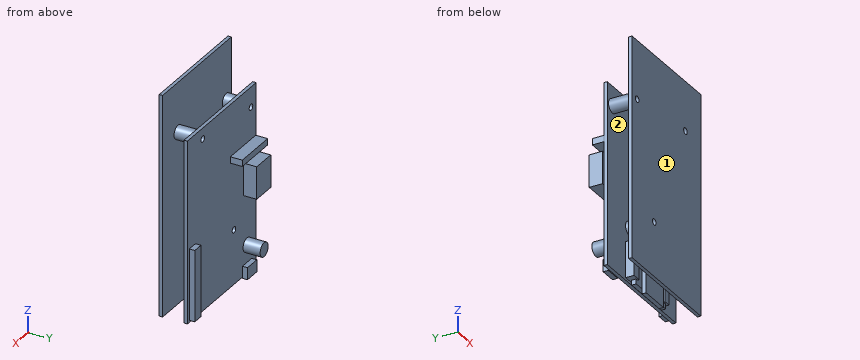
from build123d import *

# Parameters (mm, degrees)
SKETCH2_W               = 55.88
SKETCH2_H               = 85.09
FIBERGLASS_PCB_DEPTH    = 1.6
SKETCH3_W               = 7.6
SKETCH3_H               = 5.6
USB_MICRO_B_POWER_DEPTH = 2.4
SKETCH4_W               = 5
SKETCH4_H               = 33.2
BOSS_EXTRUDE3_DEPTH     = 2.6
SKETCH5_W               = 11.4
SKETCH5_H               = 15.1
BOSS_EXTRUDE4_DEPTH     = 6.15
SKETCH6_W               = 20.6
SKETCH6_H               = 2.95
BOSS_EXTRUDE5_DEPTH     = 5.6
SKETCH8_R               = 3.25
BOSS_EXTRUDE6_DEPTH     = 8
SKETCH9_W               = 28.4
SKETCH9_H               = 16.8
BOSS_EXTRUDE7_DEPTH     = 3.9
SKETCH10_W              = 24
SKETCH10_H              = 2.1
BOSS_EXTRUDE8_DEPTH     = 2.286
SKETCH11_R              = 1.45
CUT_EXTRUDE1_DEPTH      = 54.073569326
SKETCH12_R              = 3.175
BOSS_EXTRUDE9_DEPTH     = 10
SKETCH13_W              = 55.88
SKETCH13_H              = 103.09
BOSS_EXTRUDE10_DEPTH    = 1.5875
SKETCH14_R              = 1.45
CUT_EXTRUDE2_DEPTH      = 69.474424286
CUT_EXTRUDE3_DEPTH      = 0.75
SKETCH16_W              = 14.0335
SKETCH16_H              = 17.145
BOSS_EXTRUDE11_DEPTH    = 1.9685
BOSS_EXTRUDE13_REACH    = 70.474
SKETCH18_R              = 3.175
SKETCH19_R              = 1.45
CUT_EXTRUDE5_DEPTH      = 69.474424286


with BuildPart() as part:
    # Sketch2 → Fiberglass PCB (new body)
    with BuildSketch(Plane(origin=(0, 0, 0), x_dir=(1, 0, 0), z_dir=(0, 1, 0))):
        Rectangle(SKETCH2_W, SKETCH2_H)
    extrude(amount=FIBERGLASS_PCB_DEPTH)

    # Sketch3 → USB Micro-B Power (add)
    with BuildSketch(Plane(origin=(0, 1.6, 0), x_dir=(1, 0, 0), z_dir=(0, 1, 0))):
        with Locations((-20.54, 40.245)):
            Rectangle(SKETCH3_W, SKETCH3_H)
    extrude(amount=USB_MICRO_B_POWER_DEPTH)

    # Sketch4 → Boss-Extrude3 (add)
    with BuildSketch(Plane(origin=(0, 1.6, 0), x_dir=(1, 0, 0), z_dir=(0, 1, 0))):
        with Locations((23.94, 24.945)):
            Rectangle(SKETCH4_W, SKETCH4_H)
    extrude(amount=BOSS_EXTRUDE3_DEPTH)

    # Sketch5 → Boss-Extrude4 (add)
    with BuildSketch(Plane(origin=(0, 1.6, 0), x_dir=(1, 0, 0), z_dir=(0, 1, 0))):
        with Locations((-23.44, -2.505)):
            Rectangle(SKETCH5_W, SKETCH5_H)
    extrude(amount=BOSS_EXTRUDE4_DEPTH)

    # Sketch6 → Boss-Extrude5 (add)
    with BuildSketch(Plane(origin=(0, 1.6, 0), x_dir=(1, 0, 0), z_dir=(0, 1, 0))):
        with Locations((-17.26, -16.78)):
            Rectangle(SKETCH6_W, SKETCH6_H)
    extrude(amount=BOSS_EXTRUDE5_DEPTH)

    # Sketch8 → Boss-Extrude6 (add)
    with BuildSketch(Plane(origin=(0, 1.6, 0), x_dir=(1, 0, 0), z_dir=(0, 1, 0))):
        with Locations(Location((-20.54, 29.295, 0), (0, 0, 90))):
            Circle(SKETCH8_R)
    extrude(amount=BOSS_EXTRUDE6_DEPTH)

    # Sketch9 → Boss-Extrude7 (add)
    with BuildSketch(Plane.XZ):
        with Locations((1.26, -32.945)):
            Rectangle(SKETCH9_W, SKETCH9_H)
    extrude(amount=BOSS_EXTRUDE7_DEPTH)

    # Sketch10 → Boss-Extrude8 (add)
    with BuildSketch(Plane(origin=(0, 0, -41.345), x_dir=(-1, 0, 0), z_dir=(0, 0, -1))):
        with Locations((-2.097, -2.1)):
            Rectangle(SKETCH10_W, SKETCH10_H)
    extrude(amount=BOSS_EXTRUDE8_DEPTH)

    # Sketch11 → Cut-Extrude1 (cut, through all)
    with BuildSketch(Plane(origin=(0, 1.6, 0), x_dir=(1, 0, 0), z_dir=(0, 1, 0))):
        with Locations(Location((15.494, -37.465, 0), (0, 0, 270))):
            Circle(SKETCH11_R)
        with Locations(Location((-9.906, 17.145, 0), (0, 0, 270))):
            Circle(SKETCH11_R)
    extrude(amount=-CUT_EXTRUDE1_DEPTH, mode=Mode.SUBTRACT)

    # Sketch12 → Boss-Extrude9 (add)
    with BuildSketch(Plane.XZ):
        with Locations(Location((-9.906, -17.145, 0), (0, 0, 270))):
            Circle(SKETCH12_R)
        with Locations(Location((15.494, 37.465, 0), (0, 0, 270))):
            Circle(SKETCH12_R)
    extrude(amount=BOSS_EXTRUDE9_DEPTH)

    # Sketch13 → Boss-Extrude10 (add)
    with BuildSketch(Plane.XZ.offset(10)):
        with Locations((0, 9)):
            Rectangle(SKETCH13_W, SKETCH13_H)
    extrude(amount=BOSS_EXTRUDE10_DEPTH)

    # Sketch14 → Cut-Extrude2 (cut, through all)
    with BuildSketch(Plane(origin=(0, 1.6, 0), x_dir=(1, 0, 0), z_dir=(0, 1, 0))):
        with Locations(Location((-9.906, 17.145, 0), (0, 0, 270))):
            Circle(SKETCH14_R)
        with Locations(Location((15.494, -37.465, 0), (0, 0, 270))):
            Circle(SKETCH14_R)
    extrude(amount=-CUT_EXTRUDE2_DEPTH, mode=Mode.SUBTRACT)

    # Sketch15 → Cut-Extrude3 (cut)
    with BuildSketch(Plane(origin=(0, -3.9, 0), x_dir=(-1, 0, 0), z_dir=(0, -1, 0))):
        Polygon((8.7335, 41.345), (-12.412, 41.345), (-12.412, 30.12806403), (-10.16693597, 27.883), (8.7335, 27.883), align=None)
    extrude(amount=-CUT_EXTRUDE3_DEPTH, mode=Mode.SUBTRACT)

    # Sketch16 → Boss-Extrude11 (add)
    with BuildSketch(Plane.XZ.offset(3.15)):
        with Locations((1.80115, -37.4715)):
            Rectangle(SKETCH16_W, SKETCH16_H)
    extrude(amount=BOSS_EXTRUDE11_DEPTH)

    # Sketch18 → Boss-Extrude13 (add, up to next)
    with BuildSketch(Plane(origin=(0, 1.6, 0), x_dir=(1, 0, 0), z_dir=(0, 1, 0)), mode=Mode.PRIVATE) as boss_extrude13_sk1:
        with Locations(Location((-23.749, -33.1597, 0), (0, 0, 270))):
            Circle(SKETCH18_R)
    boss_extrude13_tool1 = extrude(boss_extrude13_sk1.sketch, amount=-BOSS_EXTRUDE13_REACH, mode=Mode.PRIVATE) - part.part
    add(boss_extrude13_tool1.solids().sort_by_distance((-23.749, 1.6, 33.1597))[0])

    # Sketch19 → Cut-Extrude5 (cut, through all)
    with BuildSketch(Plane(origin=(0, 1.6, 0), x_dir=(1, 0, 0), z_dir=(0, 1, 0))):
        with Locations(Location((-23.749, -33.1597, 0), (0, 0, 270))):
            Circle(SKETCH19_R)
    extrude(amount=-CUT_EXTRUDE5_DEPTH, mode=Mode.SUBTRACT)


solid = part.part
Could you check a few things on this model? Use its own coordinates, in mm. Face numbers are marked on the shaded views. Coordinates: 2 decimals unless noted, no trailing zeros. Write each loop counter-clockwise with the first axis right and the second up, starting at its lowest first coordinate (ties: lowest second). Pieces come first, ordered by that corner, then holes. Notation, with made-up numbers: (-27, -37) - (-13, -37) arc R14 ccw to (-13, -24) - close; hole circle Ø9 at (55, -13.5). An arc over 180 degrees is marked (long way). Write item = value, one per line.
1) Suppose I cut it at A-A on z = -9.5. Please give me the cut outline in (x, y), plus the area to 3 significant figures.
Result set:
outline = (-27.94, -11.59) - (27.94, -11.59) - (27.94, -10) - (-27.94, -10) - close; (-27.94, 0) - (27.94, 0) - (27.94, 1.6) - (26.44, 1.6) - (26.44, 4.2) - (21.44, 4.2) - (21.44, 1.6) - (-27.94, 1.6) - close
area = 191 mm2
2) Please list where these lines run through material, in increasing order: line 1 (Y direction, x = 19, z = 19); line 2 (Z direction, x = -24, y = -10.25) (3 decimals); line 3 (Y direction, x = -12.5, z = -38.5). Write a range as [from, to].
Result set:
line_1 = [-11.59, -10], [0, 1.6]
line_2 = [-42.545, 31.732], [34.588, 60.545]
line_3 = [-11.59, -10], [-3.9, 1.6]
3) We'd pull the mould along Y, two halves only. Please class the marked faces 1 and 2: +Y half, -Y half, draft (parallel to the pull), parting line (faces both ways), or undercut.
Result set:
face_1 = -Y half
face_2 = undercut
4) Suppose I cut it at C-C on y = -8. Please give me the cut outline in (x, z) (3 decimals), plus the area to 3 significant figures.
Result set:
outline = circle Ø6.35 at (-23.749, 33.16); circle Ø6.35 at (-9.906, -17.145); circle Ø6.35 at (15.494, 37.465); hole circle Ø2.9 at (-23.749, 33.16); hole circle Ø2.9 at (-9.906, -17.145); hole circle Ø2.9 at (15.494, 37.465)
area = 75.2 mm2
5) Suppose I cut it at D-D on z = 24. Please give me the cut outline in (x, y), plus the area to 3 significant figures.
Result set:
outline = (-27.94, -11.59) - (27.94, -11.59) - (27.94, -10) - (-27.94, -10) - close; (-27.94, 0) - (27.94, 0) - (27.94, 1.6) - (-27.94, 1.6) - close
area = 178 mm2
6) Will these pins go through, and if not, where does the flat tip stop? pin 1 Ø2.5 at (y, z) = (-2, -42) entering from -X; pin 2 Ø4.5 at (x, z) = (-19, -41) entering from +Y; pin 3 Ø10 at (x, y) = (22, 5.5) entering from -Z (3 decimals).
Result set:
pin_1 = -12.94
pin_2 = 4
pin_3 = -42.545
